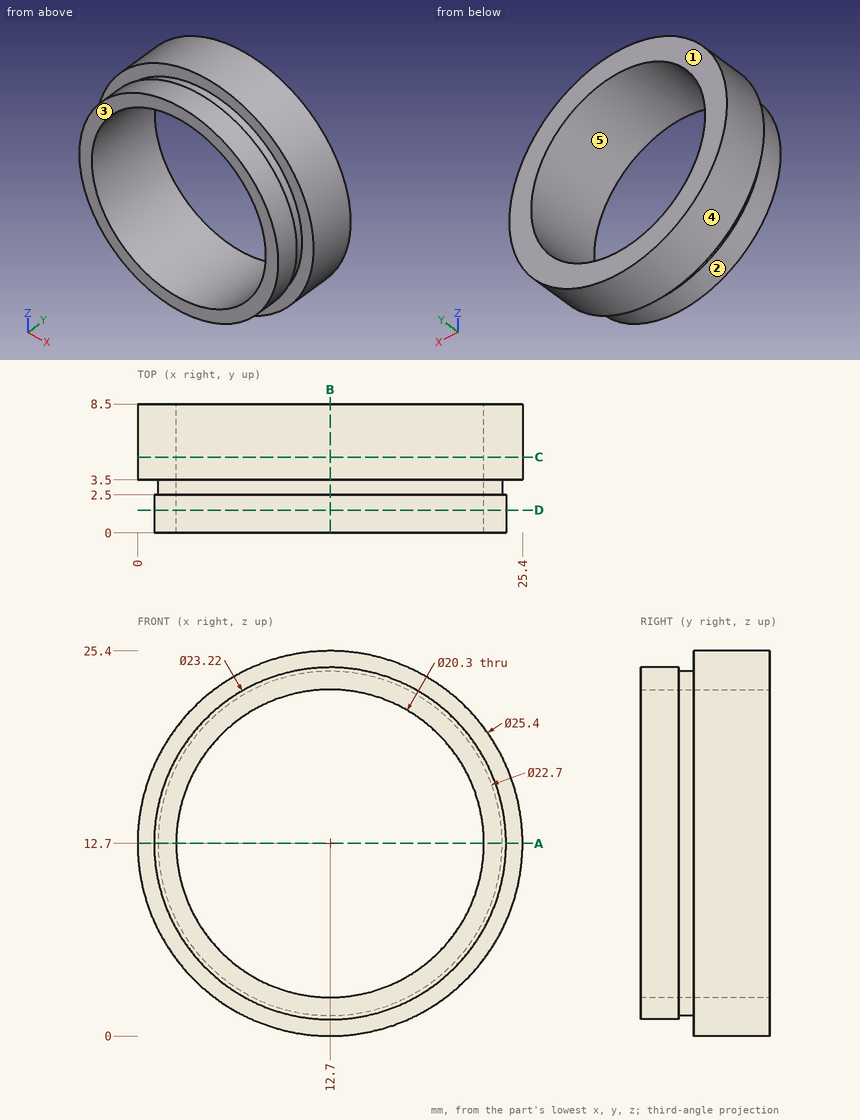
Could you check a few things on this drawing? It's one solid part, dimensions in mm from its lowest x, y, z. A direction names the side the tool comes from. Coordinates: 2 decimals unless noted, no trailing zeros. Loops run counter-clockwise (first coordinate to the right, second up) from the corner with the lowest first, then second, coordinate; pieces in that order, holes last. Notation, with made-up numbers: (75, 81.5) - (110, 81.5) arc R18 ccw to (110, 114.5) - close; hole circle Ø7 at (-18, 36). An arc over 180 degrees is marked (long way). Answer as a JSON object with one key per item and string values. Group by question number.
Item 1: If I drill on L1, parallel to Z at x = 12.7, y = 4; L2, parallel to X at y = 1.75, z = 12.5; L3, parallel to Z at x = 12.7, y = 3.25, over which ranges is the centre line in solid material (lowest first)? Write a range as from..to.
Item 2: If we section it at A-A (z = 12.7): List the corners of the cut face in (x, y) for me.
Item 3: If we mould it in two halves opening along Z, with no side actions, what happens to the marked faces 3, 4 and 5? For each: released by +Z, released by -Z, zero draft, split by the parting line, or undercut.
Item 4: On a 3-axis mill with a long thin cutter (end or side, diameter ignored), from which of +Z, -Z, +X, -X, +Y, -Y can I reach the whole of each face in a straight line? I mean the marked faces 1 and 2. Say none if no direction works.
Item 5: If we section it at B-B (x = 12.7): List the corners of the cut face in (y, z) for me, plus the area to 3 significant figures.
Item 6: For pin 1 (4 mm diameter, centred on y = 5.5, z = 16, fed in from -X); pin 2 (2 mm diameter, centred on x = 14, y = 3, fed in from -Z), each with a flat end and sliding along its axis, tell me the tip position at first contact or that it passes through.
Item 7: If we section it at D-D (y = 1.5): List the corners of the cut face in (x, z) for me, plus the area to 3 significant figures.
Item 8: If we section it at C-C (y = 5): List the corners of the cut face in (x, z) for me.
Returned:
{
 "1": {"L1": "z = 0..2.55, 22.85..25.4", "L2": "x = 1.09..2.55, 22.85..24.31", "L3": "z = 1.35..2.55, 22.85..24.05"},
 "2": {"outline": "(0, 3.5) - (1.35, 3.5) - (1.35, 2.5) - (1.09, 2.5) - (1.09, 0) - (2.55, 0) - (2.55, 8.5) - (0, 8.5) - close; (22.85, 0) - (24.31, 0) - (24.31, 2.5) - (24.05, 2.5) - (24.05, 3.5) - (25.4, 3.5) - (25.4, 8.5) - (22.85, 8.5) - close"},
 "3": {"face 3": "zero draft", "face 4": "split by the parting line", "face 5": "undercut"},
 "4": {"face 1": "+Z, -Z, +X, -X, +Y", "face 2": "-Y"},
 "5": {"outline": "(0, 1.09) - (2.5, 1.09) - (2.5, 1.35) - (3.5, 1.35) - (3.5, 0) - (8.5, 0) - (8.5, 2.55) - (0, 2.55) - close; (0, 22.85) - (8.5, 22.85) - (8.5, 25.4) - (3.5, 25.4) - (3.5, 24.05) - (2.5, 24.05) - (2.5, 24.31) - (0, 24.31) - close", "area": "35.2 mm²"},
 "6": {"pin 1": "stops at x = 0.07", "pin 2": "stops at z = 0.01"},
 "7": {"outline": "circle Ø23.22 at (12.7, 12.7); hole circle Ø20.3 at (12.7, 12.7)", "area": "99.8 mm²"},
 "8": {"outline": "circle Ø25.4 at (12.7, 12.7); hole circle Ø20.3 at (12.7, 12.7)"}
}
